from build123d import *

# Parameters (mm, degrees)
F0_W     = 152.4
F0_H     = 76.2
F1_DEPTH = 101.6
F4_DEPTH = 50.8
F5_DEPTH = 50.8
F7_DEPTH = 50.8


with BuildPart() as f1:
    # F0 (on Top) → F1 (new body)
    with BuildSketch(Plane.XY):
        with Locations((6.801184, -21.443818)):
            Rectangle(F0_W, F0_H)
    extrude(amount=F1_DEPTH)

    # F3 (on face) → F4 (cut)
    with BuildSketch(Plane.XZ.offset(59.543818)):
        Polygon((-69.398816, 101.6), (-69.398816, 76.2), (-18.598816, 76.2), (32.201184, 76.2), (83.001184, 76.2), (83.001184, 101.6), align=None)
    extrude(amount=-F4_DEPTH, mode=Mode.SUBTRACT)

    # F2 (on face) → F5 (cut)
    with BuildSketch(Plane.YZ.offset(83.001184)):
        Polygon((-59.543818, 0), (-8.743818, 76.2), (-8.743818, 101.6), (-59.543818, 101.6), align=None)
    extrude(amount=-F5_DEPTH, mode=Mode.SUBTRACT)

    # F6 (on face) → F7 (cut)
    with BuildSketch(Plane(origin=(-69.398816, 0, 0), x_dir=(0, -1, 0), z_dir=(-1, 0, 0))):
        Polygon((59.543818, 76.2), (8.743818, 76.2), (59.543818, 0), align=None)
    extrude(amount=-F7_DEPTH, mode=Mode.SUBTRACT)


solid = f1.part
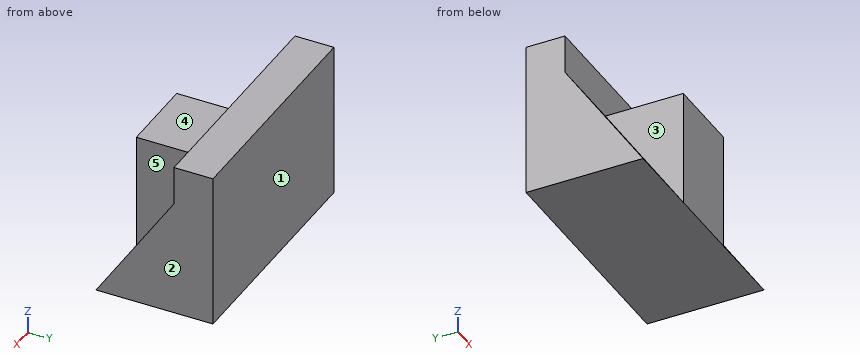
Source: CAD feature listing. Evaluate the final solid. Frame: model axes, mm. Face numbers are marked on the shaded views. A direction names the side the tool comes from. Round coordinates to 2 decimals unless told otherwise and drop trailing zeros. Write each loop counter-clockwise with the first axis right and the second up, starting at its lowest first coordinate (ties: lowest second). Pieces come first, ordered by that corner, then holes. Notation, with made-up numbers: M 10.5,46 L 55.5,46 A23 cw 55.5,56 Z; hole C -35.5,5 d4. An arc over 180 degrees is marked long. One line per item, written item: value. Start each with the question number.
Item 1: Pin query (flat end, axial travel): pin 1 (12.5 mm diameter, centred on x = 10.5, z = 92, fed in from -Y); pin 2 (12 mm diameter, centred on x = -48, y = -33, fed in from -Z); pin 3 (15 mm diameter, centred on y = -46.5, z = 34.5, fed in from -X); pin 4 (1 mm diameter, centred on x = 48.5, y = -17, fed in from +Z). Return the tip coordinate at first contact, or that it passes through.
Item 2: Section query C-C (x = -3). Return the cut outline in (y, z), plus the area to 3 significant figures.
Item 3: Section query B-B (z = 56.5). Return the cut outline in (x, y).
Item 4: Ray query, L1, parallel to Y at x = 73, z = 94.5; L2, parallel to X at y = -40.5, z = 47; L3, parallel to Z at x = -14, y = -26.5. Return the intervals inside material, ascending. Write a range as from..to.
Item 5: Section query A-A (y = -26.5). Return the cut outline in (x, z).
Item 6: Section query D-D (x = 44.5). Return the cut outline in (y, z), plus the area to 3 significant figures.
Item 7: Set-up query: the marked faces 1, 2, 3, 4 and 5. Return all of +Z, -Z, +X, -X, +Y, -Y with unobstructed straight access to the full face (end or side cutting, diameter ignored); none if empty.
Result set:
1. pin 1: stops at y = -8.74
1. pin 2: stops at z = 0
1. pin 3: stops at x = -18.6
1. pin 4: stops at z = 64.57
2. outline: M -59.54,0 L 16.66,0 L 16.66,101.6 L -8.74,101.6 L -8.74,76.2 L -59.54,76.2 Z
2. area: 6,450 mm²
3. outline: M -69.4,-21.88 L -18.6,-21.88 L -18.6,-59.54 L 32.2,-59.54 L 32.2,-21.88 L 83,-21.88 L 83,16.66 L -69.4,16.66 Z
4. L1: y = -8.74..16.66
4. L2: x = -18.6..32.2
4. L3: z = 0..76.2
5. outline: M -69.4,0 L 83,0 L 83,49.57 L 32.2,49.57 L 32.2,76.2 L -18.6,76.2 L -18.6,49.57 L -69.4,49.57 Z
6. outline: M -59.54,0 L 16.66,0 L 16.66,101.6 L -8.74,101.6 L -8.74,76.2 Z
6. area: 4,520 mm²
7. face 1: +Z, -Z, +X, -X, +Y
7. face 2: +Z, -Z, +X, +Y, -Y
7. face 3: +Z, -X, -Y
7. face 4: +Z, +X, -X, -Y
7. face 5: +Z, +X, -Y
